Part model, mm, in its own coordinate system. A direction names the side the tool comes from. Coordinates: 2 decimals unless noted, no trailing zeros. Write each loop counter-clockwise with the first axis right and the second up, starting at its lowest first coordinate (ties: lowest second). Pieces come first, ordered by that corner, then holes. Notation, with made-up numbers: (35, -17.75) -> (47, -17.75) arc R20 cw to (47, 9.25) -> close; hole circle Ø6 at (-28, -8). An arc over 180 degrees is marked (long way). Write item = value, one per line.
from build123d import *

# Parameters (mm, degrees)
BOSS_EXTRUDE1_DEPTH = 3


with BuildPart() as part:
    # Sketch1 → Boss-Extrude1 (new body)
    with BuildSketch(Plane(origin=(0, 0, 0), x_dir=(1, 0, 0), z_dir=(0, 1, 0))):
        Polygon((0, 0), (30, 0), (33, 0), (33, 5.1), (30, 5.1), (30, 10.2), (33, 10.2), (33, 15.3), (30, 15.3), (20, 15.3), (20, 12.3), (10, 12.3), (10, 15.3), (0, 15.3), align=None)
    extrude(amount=BOSS_EXTRUDE1_DEPTH)


solid = part.part
Q1. Saw through at C-C on x = 16. Give the cut face in (y, z), and give its area (3 significant figures).
Model answer:
outline = (0, -12.3) -> (3, -12.3) -> (3, 0) -> (0, 0) -> close
area = 36.9 mm²
Q2. Saw through at A-A on z = -14.5. Give the cut face in (x, y).
Model answer:
outline = (0, 0) -> (10, 0) -> (10, 3) -> (0, 3) -> close; (20, 0) -> (33, 0) -> (33, 3) -> (20, 3) -> close
Q3. Which spindle directions (+Z, -Z, +X, -X, +Y, -Y) get a long thin tool onto all of the face, cutting with end or side? Do faces 1 (the face through (15, 1, -12.3)), 2 (the face through (32, 1, -5.1)), 3 (the face through (16, 1, 0)). Say none if no direction does.
Model answer:
face_1 = -Z, +Y, -Y
face_2 = +X, +Y, -Y
face_3 = +Z, +X, -X, +Y, -Y
Q4. Mould opens along X. For faces 4 (the face through (30, 1, -8)), 5 (the face through (16, 3, -8)), 6 (the face through (20, 1, -14)) say: released by +X, released by -X, zero draft, split by the parting line, or undercut.
Model answer:
face_4 = released by +X
face_5 = zero draft
face_6 = undercut
Q5. Saw through at B-B on y = 2.15. Give the cut face in (x, z).
Model answer:
outline = (0, -15.3) -> (10, -15.3) -> (10, -12.3) -> (20, -12.3) -> (20, -15.3) -> (33, -15.3) -> (33, -10.2) -> (30, -10.2) -> (30, -5.1) -> (33, -5.1) -> (33, 0) -> (0, 0) -> close
Q6. Probe line 1 (X direction, y = 2.1, z = -12.5); line 2 (X direction, y = 2.7, z = -10); line 3 (Z direction, x = 14, y = 1.35). List the from-to ranges inside material, lowest first. Write a range as from..to.
Model answer:
line_1 = 0..10, 20..33
line_2 = 0..30
line_3 = -12.3..0
Q7. Pin check, flat tip, straight feed: pin 1 (0.9 mm diameter, centred on y = 2, z = -7.5, fed in from +X). Stop position of the tip, or through.
Model answer:
pin_1 = 30
Q8. Saw through at D-D on z = -6.5. Give the cut face in (x, y), and give its area (3 significant figures).
Model answer:
outline = (0, 0) -> (30, 0) -> (30, 3) -> (0, 3) -> close
area = 90.0 mm²
